Part model, mm, in its own coordinate system. A direction names the side the tool comes from. Give positions to 0.01 mm unless a question says otherwise; leave off trailing zeros. Answer as a JSON object with one key per item and string values.
from build123d import *

# Parameters (mm, degrees)
SKETCH2_W                 = 34.55
SKETCH2_H                 = 21.85
BOSS_EXTRUDE1_DEPTH       = 379
CUT_EXTRUDE1_DEPTH        = 379
SKETCH5_W                 = 13.55
SKETCH5_H                 = 10.4
CUT_EXTRUDE2_DEPTH        = 379
F_5_0MM_DOWEL_HOLE2_D     = 5
F_5_0MM_DOWEL_HOLE2_DEPTH = 2.25


with BuildPart() as part:
    # Sketch2 → Boss-Extrude1 (new body)
    with BuildSketch(Plane.XY):
        with Locations((17.275, 10.925)):
            Rectangle(SKETCH2_W, SKETCH2_H)
    extrude(amount=-BOSS_EXTRUDE1_DEPTH)

    # Sketch3 → Cut-Extrude1 (cut)
    with BuildSketch(Plane.XY):
        Polygon((29.55, 21.85), (17.275, 21.85), (17.275, 16.85), (27.775, 16.85), (29.55, 18.1599631), align=None)
        Polygon((34.55, 0), (34.55, 16.85), (30.55, 16.85), (30.55, 12.25), (32.55, 12.25), (32.55, 9.45), (30.25, 9.45), (30.25, 11.25), (25.85, 11.25), (25.85, 2.25), (30.25, 2.25), (30.25, 4.05), (32.55, 4.05), (32.55, 0), align=None)
    cut_extrude1 = extrude(amount=-CUT_EXTRUDE1_DEPTH, mode=Mode.SUBTRACT)

    # Mirror1: Cut-Extrude1 across plane
    add(cut_extrude1.mirror(Plane(origin=(17.275, 0, 0), x_dir=(0, 0, 1), z_dir=(1, 0, 0))), mode=Mode.SUBTRACT)

    # Sketch5 → Cut-Extrude2 (cut)
    with BuildSketch(Plane.XY):
        with Locations((17.275, 7.45)):
            Rectangle(SKETCH5_W, SKETCH5_H)
    extrude(amount=-CUT_EXTRUDE2_DEPTH, mode=Mode.SUBTRACT)

    # Ø5.0mm Dowel Hole2
    with Locations(Plane(origin=(0, 0, 0), x_dir=(-1, 0, 0), z_dir=(0, -1, 0))):
        with Locations((-17.275, 359), (-17.275, 185.4), (-17.275, 158.733333333)):
            Hole(F_5_0MM_DOWEL_HOLE2_D / 2, depth=F_5_0MM_DOWEL_HOLE2_DEPTH)


solid = part.part
1. Pin check, flat tips, straight feed: P1, Ø8, axis at y = 2.5, z = -256.5, coming from the +X side; P2, Ø2.5, axis at y = 8.5, z = -195.5, coming from the -X side; P3, Ø5, axis at x = 15, y = 9, coming from the -Z side; P4, Ø4.5, axis at x = 17.275, z = -185.4, coming from the +Y side. Stop position of each tip, or through.
Worked answers:
{"P1": "stops at x = 32.55", "P2": "stops at x = 2", "P3": "passes through", "P4": "stops at y = 16.85"}
2. Probe line 1 along X through (y, z) = (10, -289.5); line 2 along X through (y, z) = (1.15, -359) (3 decimals); line 3 along Y through (x, z) = (26.5, -68.5). List the from-to ranges inside material, lowest first.
Worked answers:
{"line 1": "x = 2 to 4.3, 8.7 to 10.5, 24.05 to 25.85, 30.25 to 32.55", "line 2": "x = 2 to 14.775, 19.775 to 32.55", "line 3": "y = 0 to 2.25, 11.25 to 16.85"}
3. Which spindle directions (+Z, -Z, +X, -X, +Y, -Y) get a long thin tool onto all of the face, cutting with end or side? Do faces 1 (the flat face through (17, 14, -379)), 2 (the flat face through (17, 12.65, -187)). Say none if no direction does.
Worked answers:
{"face 1": "-Z, +X, -X, +Y, -Y", "face 2": "+Z, -Z"}
4. Two-plate mould, pull along Y, no slides. Class faces 3 (the flat face through (14, 0, -187)), 4 (the flat face through (17, 16.85, -187)), 5 (the flat face through (24.05, 7, -187)), 6 (the flat face through (17, 14, 0)): +Y half, -Y half, draft (parallel to the pull), parting line (faces both ways), or undercut.
Worked answers:
{"face 3": "-Y half", "face 4": "+Y half", "face 5": "undercut", "face 6": "draft"}
